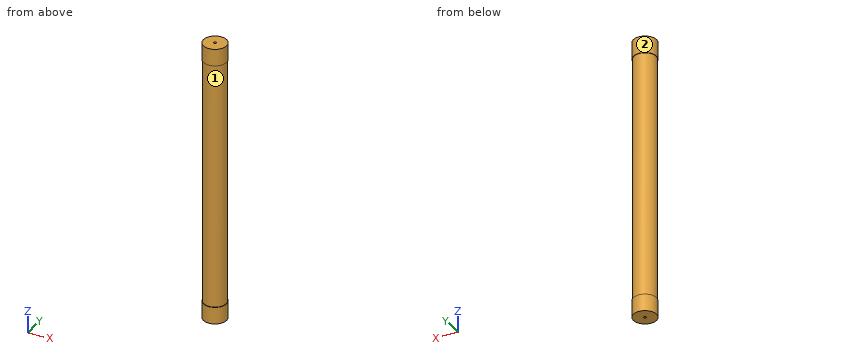
from build123d import *

# Parameters (mm, degrees)
F0_R     = 2.5
F1_DEPTH = 27.836615
F2_R     = 2.6
F2_R_2   = 2.5
F3_DEPTH = 3.813385
F4_R     = 2.6
F4_R_2   = 2.5
F5_DEPTH = 3.813385
F6_R     = 0.3
F7_DEPTH = 0.1
F8_R     = 0.3
F9_DEPTH = 0.1


with BuildPart() as f1:
    # F0 (on Top) → F1 (new body, symmetric)
    with BuildSketch(Plane.XY):
        Circle(F0_R)
    extrude(amount=F1_DEPTH, both=True)

    # F2 (on face) → F3 (join)
    with BuildSketch(Plane.XY.offset(27.836615)):
        Circle(F2_R)
        Circle(F2_R_2, mode=Mode.SUBTRACT)
        Circle(F2_R_2)
    extrude(amount=F3_DEPTH)

    # F4 (on face) → F5 (join)
    with BuildSketch(Plane(origin=(0, 0, -27.836615), x_dir=(1, 0, 0), z_dir=(0, 0, -1))):
        Circle(F4_R)
        Circle(F4_R_2, mode=Mode.SUBTRACT)
        Circle(F4_R_2)
    extrude(amount=F5_DEPTH)

    # F6 (on face) → F7 (join)
    with BuildSketch(Plane(origin=(0, 0, -31.65), x_dir=(1, 0, 0), z_dir=(0, 0, -1))):
        Circle(F6_R)
    extrude(amount=F7_DEPTH)

    # F8 (on face) → F9 (join)
    with BuildSketch(Plane.XY.offset(31.65)):
        Circle(F8_R)
    extrude(amount=F9_DEPTH)


solid = f1.part
For this review, take the finished solid that the model builds, in its own axes (mm). Face numbers are marked on the shaded views. Give positions to 0.01 mm unless a question says otherwise; leave off trailing zeros. Order: outer loops, then holes, each group sorted by start corner. A loop starts at its lowest first (then second) coordinate and runs counter-clockwise, first axis right, second up. Notation, with made-up numbers: M 73.25,-30.5 L 120.25,-30.5 A20 ccw 120.25,-24.5 Z; hole C 62.5,-32 d5. An arc over 180 degrees is marked long. Answer in a Markdown table with one row per item. Add a question column.
(1) Mouldability with a two-part tool opening along Z and no side actions: class the marked faces 1 and 2 as +Z half, -Z half, draft (parallel to the pull), parting line (faces both ways), or undercut.
(2) For pin 1 (1 mm diameter, centred on y = -1, z = 24.5, fed in from -X); pin 2 (1.5 mm diameter, centred on x = -1.5, z = 5.5, fed in from +Y); pin 3 (1 mm diameter, centred on x = -1.5, z = 21, fed in from -Y), all flat-tipped, find the tip position at first contact; note any pin that passes through.
(3) Consider section A-A on y = 1.8. State the section outline as (x, z) points.
(4) Consider section B-B on z = -14. State the section outline as (x, y) points, and give its area (3 significant figures).
(5) Consider section C-C on x = 0.85. State the section outline as (y, z) points, and give its area (3 significant figures).
(6) Wall thickness on probe 1 along Z at (x, y) = (-0.75, -1.55); probe 2 along Y at (x, z) = (0, -11.5); probe 3 along X at (y, z) = (-1, -13.5): over which ranges is each line inside the solid? List them lowest first. Write a range as [from, to].
Evaluation:
| question | item | result |
|---|---|---|
| 1 | face 1 | undercut |
| 1 | face 2 | draft |
| 2 | pin 1 | stops at x = -2.45 |
| 2 | pin 2 | stops at y = 2.38 |
| 2 | pin 3 | stops at y = -2.29 |
| 3 | outline | M -1.88,-31.65 L 1.88,-31.65 L 1.88,-27.84 L 1.73,-27.84 L 1.73,27.84 L 1.88,27.84 L 1.88,31.65 L -1.88,31.65 L -1.88,27.84 L -1.73,27.84 L -1.73,-27.84 L -1.88,-27.84 Z |
| 4 | outline | C 0,0 d5 |
| 4 | area | 19.6 mm^2 |
| 5 | outline | M -2.46,-31.65 L 2.46,-31.65 L 2.46,-27.84 L 2.35,-27.84 L 2.35,27.84 L 2.46,27.84 L 2.46,31.65 L -2.46,31.65 L -2.46,27.84 L -2.35,27.84 L -2.35,-27.84 L -2.46,-27.84 Z |
| 5 | area | 299 mm^2 |
| 6 | probe 1 | z = [-31.65, 31.65] |
| 6 | probe 2 | y = [-2.5, 2.5] |
| 6 | probe 3 | x = [-2.29, 2.29] |
